```python
from build123d import *

# Parameters (mm, degrees)
SKETCH2_W         = 4
SKETCH2_H         = 8.15
BOTTOM_DEPTH      = 2.7
SKETCH3_R         = 2
TOP_DEPTH         = 6.9
SKETCH4_R         = 1.25
TENDON_HOLE_DEPTH = 13.5


with BuildPart() as part:
    # Sketch2 → bottom (new body)
    with BuildSketch(Plane(origin=(0, 0, 0), x_dir=(1, 0, 0), z_dir=(0, 1, 0))):
        Rectangle(SKETCH2_W, SKETCH2_H)
    extrude(amount=-BOTTOM_DEPTH)

    # Sketch3 → top (add)
    with BuildSketch(Plane(origin=(0, 0, 0), x_dir=(1, 0, 0), z_dir=(0, 1, 0))):
        with Locations((0, -1.175)):
            Circle(SKETCH3_R)
    extrude(amount=TOP_DEPTH)

    # Sketch4 → tendon hole (cut)
    with BuildSketch(Plane.XY.offset(4.075)):
        with Locations((0, 3.45)):
            Circle(SKETCH4_R)
    extrude(amount=-TENDON_HOLE_DEPTH, mode=Mode.SUBTRACT)


solid = part.part
```
Read the model definition and answer for the solid it produces. Units are mm, in the model's axes. Give positions to 0.01 mm unless a question says otherwise; leave off trailing zeros. Write each loop counter-clockwise with the first axis right and the second up, starting at its lowest first coordinate (ties: lowest second). Pieces come first, ordered by that corner, then holes. Notation, with made-up numbers: (3, -10.5) - (52, -10.5) arc R10 cw to (52, -1.5) - close; hole circle Ø10 at (-35, -39). An arc over 180 degrees is marked (long way). Write item = value, one per line. Start each with the question number.
Item 1: This flat-tipped pin is pushed along its axis until it touches: P1, Ø1.5, axis at x = -0.5, y = 3, coming from the +Z side. Where does it stop, or does it pass through?
Item 2: Find section B-B (z = 0.5). Give the vertices of the cut face in (x, y).
Item 3: Find the intervals of material crossed by probe 1 along Y at (x, z) = (0, 0.1); probe 2 along Y at (x, z) = (-0.2, -2.75); probe 3 along X at (y, z) = (3.45, 0.1), in increasing order. Write a range as [from, to].
Item 4: Find section C-C (y = 3). Give the vertices of the cut face in (x, z) (3 decimals), then the cut area to 3 significant figures.
Item 5: Find section A-A (x = 0). Give the vertices of the cut face in (y, z) (3 decimals), then the cut area to 3 significant figures.
Item 6: The mould has two halves that part along X. Classify faces 1 (the flat face through (2, -1, 0)), 2 (the flat face through (0, 0, 3.6)), 3 (the cylindrical face through (0.672, 4.504, 1.203)), 4 (the cylindrical face through (-1.47, 3.4, -0.18)): +X half, -X half, draft (parallel to the pull), parting line (faces both ways), or undercut.
Item 7: Find section D-D (x = -1). Give the vertices of the cut face in (y, z) (3 decimals), then the cut area to 3 significant figures.
Response:
q1.P1 = 3.14
q2.outline = (-2, -2.7) - (2, -2.7) - (2, 0) - (1.88, 0) - (1.88, 6.9) - (-1.88, 6.9) - (-1.88, 0) - (-2, 0) - close; hole circle Ø2.5 at (0, 3.45)
q3.probe_1 = [-2.7, 2.2], [4.7, 6.9]
q3.probe_2 = [-2.7, 0]
q3.probe_3 = [-1.69, -1.25], [1.25, 1.69]
q4.outline = (-1.166, -0.45) - (-1.166, 2.8) arc R2 ccw to start; (1.166, -0.45) arc R2 ccw to (1.166, 2.8) - close
q4.area = 3.80 mm²
q5.outline = (-2.7, -4.075) - (0, -4.075) - (0, -0.825) - (2.2, -0.825) - (2.2, 3.175) - (0, 3.175) - (0, 4.075) - (-2.7, 4.075) - close; (4.7, -0.825) - (6.9, -0.825) - (6.9, 3.175) - (4.7, 3.175) - close
q5.area = 39.6 mm²
q6.face_1 = +X half
q6.face_2 = draft
q6.face_3 = undercut
q6.face_4 = parting line
q7.outline = (-2.7, -4.075) - (0, -4.075) - (0, -0.557) - (2.7, -0.557) - (2.7, 2.907) - (0, 2.907) - (0, 4.075) - (-2.7, 4.075) - close; (4.2, -0.557) - (6.9, -0.557) - (6.9, 2.907) - (4.2, 2.907) - close
q7.area = 40.7 mm²
